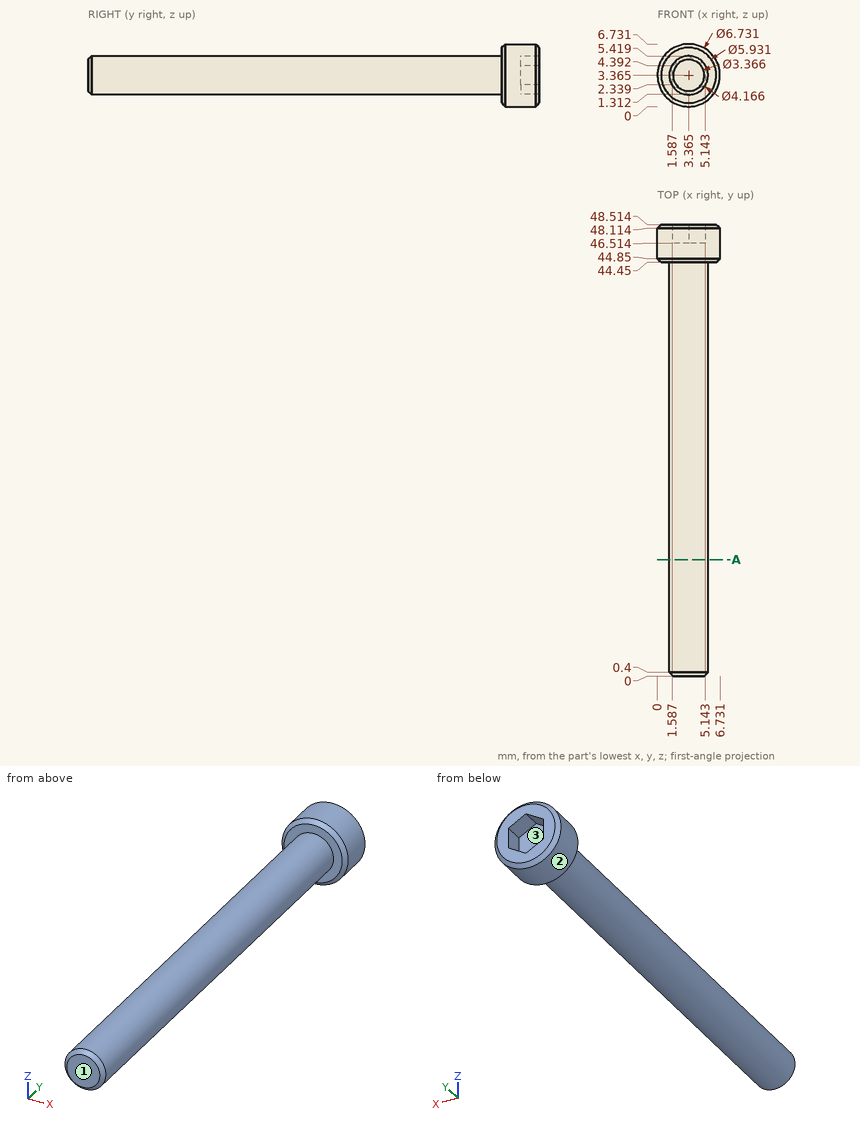
Check sheet for the drawn part. Datum: minimum x, y, z corner. Units: mm. Coordinates: 2 decimals unless noted, no trailing zeros. Order: outer loops, then holes, each group sorted by start corner. A loop starts at its lowest first (then second) coordinate and runs counter-clockwise, first axis right, second up. Notation, with made-up numbers: M 33.25,-21 L 51.25,-21 A4 cw 51.25,-14 Z; hole C 1.5,3 d6. An arc over 180 degrees is marked long. One line per question, with ' | ' between items. Start each with the question number.
Item 1: Material ranges on line 1 (Z direction, x = 3.25, y = 11) (1 decimal); line 2 (Y direction, x = 2.5, z = 3) (1 decimal); line 3 (X direction, y = 10.5, z = 3.75), recorded low to high.
Item 2: Sectioned sample at A-A on y = 12.5. Record the cut outline in (x, z) (1 decimal), and give its area (3 significant figures).
Item 3: Mould release check, pull along X, two halves, no side actions. Record for the marked faces 1, 2 and 3: pulls with the +X half, pulls with the -X half, needs draft (parallel to the pull), parting line crosses it, or undercut.
Item 4: Gauge pin test, flat ends, axial feed: P1, Ø1.5, axis at x = 3, y = 36.5, coming from the -Z side; P2, Ø1, axis at x = 5.5, z = 4, coming from the -Y side (1 decimal); P3, Ø0.6, axis at y = 47, z = 4, coming from the -X side. Record the tip position at first contact, or that the pin passes through.
Answer below:
1) line 1: z = 1.3 to 5.4 | line 2: y = 0 to 46.5 | line 3: x = 1.32 to 5.41
2) outline: C 3.4,3.4 d4.2 | area: 13.6 mm^2
3) face 1: needs draft | face 2: parting line crosses it | face 3: undercut
4) P1: stops at z = 1.28 | P2: stops at y = 0 | P3: stops at x = 0.02
